```python
from build123d import *

# Parameters (mm, degrees)
SKETCH1_R          = 34.925
EXTRUDE1_DEPTH     = 12.7
SKETCH2_R          = 8.636
CUT_EXTRUDE1_DEPTH = 51.998051433
SKETCH3_R          = 3.3655
CUT_EXTRUDE2_DEPTH = 12.7
CIRPATTERN1_COUNT  = 6
SKETCH5_R          = 2.1844
CUT_EXTRUDE4_DEPTH = 51.998051433
CIRPATTERN2_COUNT  = 6


with BuildPart() as part:
    # Sketch1 → Extrude1 (new body)
    with BuildSketch(Plane(origin=(0, 0, 0), x_dir=(1, 0, 0), z_dir=(0, 1, 0))):
        with Locations(Location((0, 0, 0), (0, 0, 270))):
            Circle(SKETCH1_R)
    extrude(amount=EXTRUDE1_DEPTH)

    # Sketch2 → Cut-Extrude1 (cut, through all)
    with BuildSketch(Plane(origin=(0, 0, 0), x_dir=(1, 0, 0), z_dir=(0, 1, 0))):
        with Locations(Location((0, 0, 0), (0, 0, 270))):
            Circle(SKETCH2_R)
    extrude(amount=CUT_EXTRUDE1_DEPTH, mode=Mode.SUBTRACT)

    # Sketch3 → Cut-Extrude2 (cut)
    with BuildSketch(Plane(origin=(0, 0, 0), x_dir=(1, 0, 0), z_dir=(0, 1, 0))):
        with Locations(Location((0, 29.337, 0), (0, 0, 270))):
            Circle(SKETCH3_R)
    cut_extrude2 = extrude(amount=CUT_EXTRUDE2_DEPTH, mode=Mode.SUBTRACT)

    # CirPattern1: Cut-Extrude2 ×6 about axis
    cirpattern1_axis = Axis((0, 0, 0), (0, 1, 0))
    for i in range(1, CIRPATTERN1_COUNT):
        add(cut_extrude2.rotate(cirpattern1_axis, i * 360 / CIRPATTERN1_COUNT), mode=Mode.SUBTRACT)

    # Sketch5 → Cut-Extrude4 (cut, through all)
    with BuildSketch(Plane(origin=(0, 0, 0), x_dir=(1, 0, 0), z_dir=(0, 1, 0))):
        with Locations(Location((0, 13.462, 0), (0, 0, 270))):
            Circle(SKETCH5_R)
    cut_extrude4 = extrude(amount=CUT_EXTRUDE4_DEPTH, mode=Mode.SUBTRACT)

    # CirPattern2: Cut-Extrude4 ×6 about axis
    cirpattern2_axis = Axis((0, 0, 0), (0, 1, 0))
    for i in range(1, CIRPATTERN2_COUNT):
        add(cut_extrude4.rotate(cirpattern2_axis, i * 360 / CIRPATTERN2_COUNT), mode=Mode.SUBTRACT)


solid = part.part
```
Geometry check sheet. Reference: the model listing, model coordinates, mm. Give positions to 0.01 mm unless a question says otherwise; leave off trailing zeros. Order: outer loops, then holes, each group sorted by start corner. A loop starts at its lowest first (then second) coordinate and runs counter-clockwise, first axis right, second up. Notation, with made-up numbers: (27.25, 79) - (35.25, 79) arc R19 cw to (35.25, 103) - close; hole circle Ø9 at (-5, 46.5). An arc over 180 degrees is marked (long way). Answer in a Markdown table with one row per item. Add a question column.
Q1. Cross-section at D-D, the plane y = 9. Count the separate pieces of the cut face and the enclosed holes in it, then the cut area to 3 significant figures.
Q2. Cross-section at C-C, the plane x = 26. Enter the section's corners in (y, z).
Q3. Cross-section at B-B, the plane x = 0. Enter the section's corners in (y, z) (1 decimal).
Q4. Mould release check, pull along X, two halves, no side actions. Record for faces 1 (the flat face through (-7, 0, 7)), 2 (the cylindrical face through (-34.094, 6.261, -7.571)), 3 (the cylindrical face through (11.56, 6.26, -4.55)): pulls with the +X half, pulls with the -X half, needs draft (parallel to the pull), parting line crosses it, or undercut.
Q5. Cross-section at A-A, the plane z = 0. Enter the section's corners in (x, y) (3 decimals).
Q6. Material ranges on probe 1 along Z at (x, y) = (25.5, 11.75); probe 2 along X at (y, z) = (8.25, 15); probe 3 along X at (y, z) = (8.25, 5), recorded low to high. Write a range as from..to.
Q7. Gauge pin test, flat ends, axial feed: pin 1 (2 mm diameter, centred on x = -26, y = 6.5, fed in from -Z); pin 2 (5 mm diameter, centred on y = 5.5, z = -24.5, fed in from +X); pin 3 (1 mm diameter, centred on y = 7.5, z = 4.5, fed in from +X). Record the tip position at first contact, or that the pin passes through.
Check values:
| question | item | result |
|---|---|---|
| 1 | separate pieces | 1 |
| 1 | enclosed holes | 13 |
| 1 | area | 3,290 mm^2 |
| 2 | outline | (0, -23.32) - (12.7, -23.32) - (12.7, -17.98) - (0, -17.98) - close; (0, -11.36) - (12.7, -11.36) - (12.7, 11.36) - (0, 11.36) - close; (0, 17.98) - (12.7, 17.98) - (12.7, 23.32) - (0, 23.32) - close |
| 3 | outline | (0, -34.9) - (12.7, -34.9) - (12.7, -32.7) - (0, -32.7) - close; (0, -26) - (12.7, -26) - (12.7, -15.6) - (0, -15.6) - close; (0, -11.3) - (12.7, -11.3) - (12.7, -8.6) - (0, -8.6) - close; (0, 8.6) - (12.7, 8.6) - (12.7, 11.3) - (0, 11.3) - close; (0, 15.6) - (12.7, 15.6) - (12.7, 26) - (0, 26) - close; (0, 32.7) - (12.7, 32.7) - (12.7, 34.9) - (0, 34.9) - close |
| 4 | face 1 | needs draft |
| 4 | face 2 | parting line crosses it |
| 4 | face 3 | undercut |
| 5 | outline | (-34.925, 0) - (-8.636, 0) - (-8.636, 12.7) - (-34.925, 12.7) - close; (8.636, 0) - (34.925, 0) - (34.925, 12.7) - (8.636, 12.7) - close |
| 6 | probe 1 | z = -23.86..-18.03, -11.3..11.3, 18.03..23.86 |
| 6 | probe 2 | x = -31.54..-28.76, -22.06..-1.55, 1.55..22.06, 28.76..31.54 |
| 6 | probe 3 | x = -34.57..-12.99, -10.33..-7.04, 7.04..10.33, 12.99..34.57 |
| 7 | pin 1 | stops at z = -24.39 |
| 7 | pin 2 | stops at x = 27.12 |
| 7 | pin 3 | stops at x = 34.7 |
